```python
from build123d import *

# Parameters (mm, degrees)
SKETCH005_W     = 500
SKETCH005_H     = 290
PAD005_DEPTH    = 5
POCKET_DEPTH    = 1
POCKET001_DEPTH = 1


with BuildPart() as part:
    # Sketch005 → Pad005 (new body)
    with BuildSketch(Plane.XY):
        Rectangle(SKETCH005_W, SKETCH005_H)
    extrude(amount=PAD005_DEPTH)

    # Sketch006 (on Face5 of Pad005) → Pocket (cut)
    with BuildSketch(Plane(origin=(0, 0, 0), x_dir=(1, 0, 0), z_dir=(0, 0, -1))):
        with BuildLine():
            Line((-230, 105), (47, 105))
            ThreePointArc((57, 95), (54.071068, 102.071068), (47, 105))
            Line((57, -95), (57, 95))
            ThreePointArc((47, -105), (54.071068, -102.071068), (57, -95))
            Line((-230, -105), (47, -105))
            ThreePointArc((-240, -95), (-237.071068, -102.071068), (-230, -105))
            Line((-240, -95), (-240, 95))
            ThreePointArc((-230, 105), (-237.071068, 102.071068), (-240, 95))
        make_face()
    extrude(amount=-POCKET_DEPTH, mode=Mode.SUBTRACT)

    # Sketch007 (on Face4 of Pocket) → Pocket001 (cut)
    with BuildSketch(Plane(origin=(0, 0, 0), x_dir=(1, 0, 0), z_dir=(0, 0, -1))):
        with BuildLine():
            Line((67, 105), (195, 105))
            ThreePointArc((205, 95), (202.071068, 102.071068), (195, 105))
            Line((205, -95), (205, 95))
            ThreePointArc((195, -105), (202.071068, -102.071068), (205, -95))
            Line((67, -105), (195, -105))
            ThreePointArc((57, -95), (59.928932, -102.071068), (67, -105))
            Line((57, -95), (57, 95))
            ThreePointArc((67, 105), (59.928932, 102.071068), (57, 95))
        make_face()
    extrude(amount=-POCKET001_DEPTH, mode=Mode.SUBTRACT)


with BuildPart() as part_1:
    # Body005 placement: moved
    add(part.part.moved(Location((0, 0, 105))))


solid = part_1.part
```
Can you work these out from the model? Positions are in its coordinate system, mm. A direction names the side the tool comes from. Coordinates: 2 decimals unless noted, no trailing zeros. Loops run counter-clockwise (first coordinate to the right, second up) from the corner with the lowest first, then second, coordinate; pieces in that order, holes last. Notation, with made-up numbers: M -2,0.25 L 26,0.25 A17 cw 26,10.25 Z; hole C 53,58.25 d10. An arc over 180 degrees is marked long. Put each result on its own line as item: value. Start each with the question number.
(1) I need wall thicknesses on probe 1 along Y at (x, z) = (-91, 105.35); probe 2 along Z at (x, y) = (-109, 53.5). Which ranges of each line are inside material? Lowest first, please.
(2) Which directions (+Z, -Z, +X, -X, +Y, -Y) give clear straight access to the entire face, cutting with the end or side of a thin tool? Please do faces 1 (the face through (201.99, 102.15, 105.49)), 2 (the face through (17, -107, 105)).
(3) Imagine slicing it at B-B on y = 49. List the corners of the cut face in (x, z) for me, and give its area (4 significant figures).
(4) Will this pin go through, and if not, where does the flat tip stop? pin 1 Ø1.5 at (x, y) = (23.5, -21.5) entering from -Z.
(5) We'd pull the mould along X, two halves only. Please class faces 3 (the face through (53.99, 102.15, 105.49)), 4 (the face through (-3, 2, 110)): +X half, -X half, draft (parallel to the pull), parting line (faces both ways), or undercut.
(6) Imagine slicing it at A-A on x = -136. List the corners of the cut face in (y, z) for me, and give its area (3 significant figures).
Worked answers:
1. probe 1: y = -145 to -105, 105 to 145
1. probe 2: z = 106 to 110
2. face 1: -Z
2. face 2: -Z, +X, -X, +Y, -Y
3. outline: M -250,105 L -240,105 L -240,106 L 205,106 L 205,105 L 250,105 L 250,110 L -250,110 Z
3. area: 2,055 mm2
4. pin 1: stops at z = 106
5. face 3: undercut
5. face 4: draft
6. outline: M -145,105 L -105,105 L -105,106 L 105,106 L 105,105 L 145,105 L 145,110 L -145,110 Z
6. area: 1,240 mm2
